Here's how the part is built. I have some questions about the finished solid (model axes, mm). A direction names the side the tool comes from. Give positions to 0.01 mm unless a question says otherwise; leave off trailing zeros. Write each loop counter-clockwise with the first axis right and the second up, starting at its lowest first coordinate (ties: lowest second). Pieces come first, ordered by that corner, then holes. Notation, with made-up numbers: M 19.25,57.5 L 60.25,57.5 A13 ccw 60.25,61.5 Z; hole C -3.75,68 d3. An arc over 180 degrees is marked long. Answer as CSV lines item,"result". Start each with the question number.
Q1. Thinking about a two-plate mould opening in X: for faces 5 (the flat face through (10, 39, 0)), 6 (the flat face through (-32, 79, 0)), 7 (the cylindrical face through (-22.85, 75.99, 0.07)), 8 (the cylindrical face through (26.014, 14.703, 0.07)), which applies, +X half, -X half, draft (parallel to the pull), parting line (faces both ways), or undercut?
Q2. If I drill on line 1 along X through (y, z) = (66.5, -0.5); line 2 along Y through (x, z) = (30.05, 0); line 3 along Y through (x, z) = (-40, -3), over which ranges is the centre line in solid material (lowest first)?
Q3. On a 3-axis mill with a long thin cutter (end or side, diameter ignored), from which of +Z, -Z, +X, -X, +Y, -Y can I reach the whole of each face in a straight line? I mean faces 1 (the flat face through (-10, 39, 0)), 2 (the cylindrical face through (22.85, 75.99, 0.07)), 3 (the cylindrical face through (-26.014, 14.703, 0.07)), 4 (the cylindrical face through (30.94, 83.34, -0.37)). Say none if no direction works.
Q4. Suppose I cut it at C-C (x = 3.5). Write out the boundary of the cut face in (y, z).
Q5. Suppose I cut it at B-B (z = -3.5). Write out the boundary of the cut face in (x, y).
Q6. For pin 1 (3 mm diameter, centred on y = 48.5, z = 2, fed in from +X); pin 2 (5 mm diameter, centred on y = 84, z = 2, fed in from +X); pin 3 (3 mm diameter, centred on y = 65.5, z = -2, fed in from -X), each with a flat end and sliding along its axis, tell me the tip position at first contact or that it passes through.
Q7. Suppose I cut it at A-A (y = 43). Write out the boundary of the cut face in (x, z).
```python
from build123d import *

# Parameters (mm, degrees)
SKETCH1_R                = 2.5
SKETCH1_R_2              = 4
BOSS_EXTRUDE1_DEPTH      = 5
FILLET1_R                = 1
M3_CLEARANCE_HOLE1_D     = 3.4
M3_CLEARANCE_HOLE1_DEPTH = 5
M3_CLEARANCE_HOLE1_TIP   = 1.021463052


with BuildPart() as part:
    # Sketch1 → Boss-Extrude1 (new, symmetric)
    with BuildSketch(Plane.XY):
        with BuildLine():
            ThreePointArc((10, 9), (7.071067812, 1.928932188), (0, -1))
            Line((0, -1), (0, -9))
            Line((0, -9), (40, -9))
            ThreePointArc((40, -9), (49, 0), (40, 9))
            ThreePointArc((40, 9), (25.857864376, 14.857864376), (20, 29))
            Line((20, 29), (20, 69))
            ThreePointArc((20, 69), (22.928932188, 76.071067812), (30, 79))
            Line((30, 79), (33.47, 79))
            Line((33.47, 79), (33.47, 91))
            Line((33.47, 91), (10, 91))
            Line((10, 91), (0, 82.776266062))
            Line((0, 82.776266062), (0, 79))
            ThreePointArc((0, 79), (7.071067812, 76.071067812), (10, 69))
            Line((10, 69), (10, 9))
        make_face()
        with Locations((10, 82.776266062)):
            Circle(SKETCH1_R, mode=Mode.SUBTRACT)
        with Locations((40, 0)):
            Circle(SKETCH1_R_2, mode=Mode.SUBTRACT)
    boss_extrude1 = extrude(amount=BOSS_EXTRUDE1_DEPTH, both=True)

    # Mirror1: Boss-Extrude1 across plane
    add(boss_extrude1.mirror(Plane(origin=(0, 0, 5), x_dir=(0, 0, 1), z_dir=(-1, 0, 0))))

    # Fillet1
    fillet1_edges = [part.edges().sort_by_distance(p)[0] for p in [
        (0, 82.776266062, 0),
        (10, 91, 0),
        (-10, 91, 0),
    ]]
    fillet(fillet1_edges, radius=FILLET1_R)

    # M3 Clearance Hole1
    with Locations(Plane(origin=(33.47, 0, 0), x_dir=(0, 0, -1), z_dir=(1, 0, 0))):
        with Locations((0, 85)):
            Hole(M3_CLEARANCE_HOLE1_D / 2, depth=M3_CLEARANCE_HOLE1_DEPTH)
            with Locations((0, 0, -(M3_CLEARANCE_HOLE1_DEPTH + M3_CLEARANCE_HOLE1_TIP / 2))):  # 118° drill point
                Cone(0, M3_CLEARANCE_HOLE1_D / 2, M3_CLEARANCE_HOLE1_TIP, mode=Mode.SUBTRACT)


solid = part.part
```
Resolved:
1,face 5,"undercut"
1,face 6,"draft"
1,face 7,"-X half"
1,face 8,"+X half"
2,line 1,"-20 to -10, 10 to 20"
2,line 2,"-9 to 11.65, 79 to 83.3, 86.7 to 91"
2,line 3,"-9 to -4, 4 to 9"
3,face 1,"+Z, -Z"
3,face 2,"+Z, -Z, +X"
3,face 3,"+Z, -Z, -X"
3,face 4,"+X"
4,outline,"M -9,-5 L -0.37,-5 L -0.37,5 L -9,5 Z; M 78.37,-5 L 85.65,-5 L 85.65,5 L 78.37,5 Z"
5,outline,"M -40,-9 L 40,-9 A9 ccw 40,9 A20 cw 20,29 L 20,69 A10 cw 30,79 L 33.47,79 L 33.47,91 L 10.36,91 A1 ccw 9.72,90.77 L 0.64,83.3 A1 cw -0.64,83.3 L -9.72,90.77 A1 ccw -10.36,91 L -33.47,91 L -33.47,79 L -30,79 A10 cw -20,69 L -20,29 A20 cw -40,9 A9 ccw Z; hole C -40,0 d8; hole C -10,82.78 d5; hole M -10,9 A10 ccw 10,9 L 10,69 A10 ccw -10,69 Z; hole C 10,82.78 d5; hole C 40,0 d8"
6,pin 1,"x = 20"
6,pin 2,"x = 33.47"
6,pin 3,"x = -20"
7,outline,"M -20,-5 L -10,-5 L -10,5 L -20,5 Z; M 10,-5 L 20,-5 L 20,5 L 10,5 Z"
